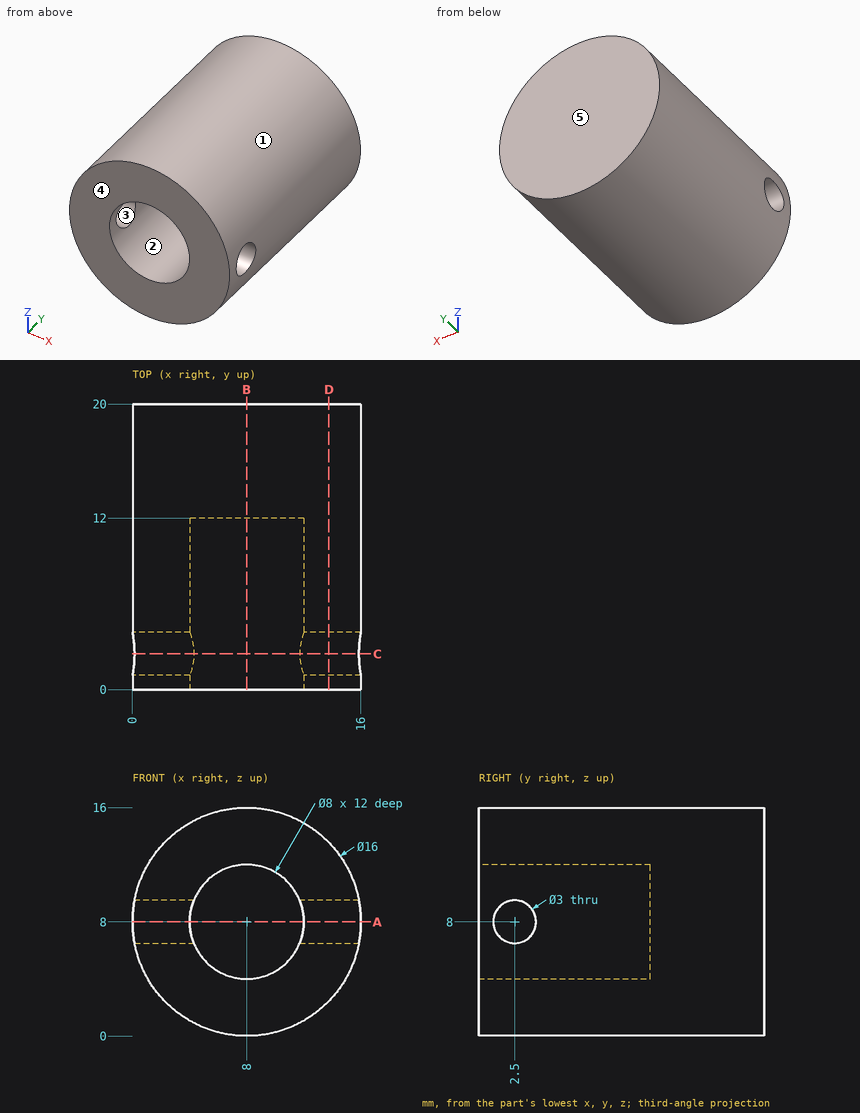
Here's the drawing with two shaded views (mm, measured from the low corner). I have some questions. A direction names the side the tool comes from. Give positions to 0.01 mm unless a question says otherwise; leave off trailing zeros. Loops run counter-clockwise (first coordinate to the right, second up) from the corner with the lowest first, then second, coordinate; pieces in that order, holes last. Notation, with made-up numbers: (-17, 58) -> (-8, 58) arc R26 ccw to (-8, 90) -> close; hole circle Ø8 at (-36, 20.25). An arc over 180 degrees is marked (long way). One line per item, written item: value.
Q1. Suppose I cut it at C-C on y = 2.5. Please give me the cut outline in (x, z).
Answers follow:
outline: (0.14, 6.5) arc R8 ccw to (15.86, 6.5) -> (11.71, 6.5) arc R4 cw to (4.29, 6.5) -> close; (0.14, 9.5) -> (4.29, 9.5) arc R4 cw to (11.71, 9.5) -> (15.86, 9.5) arc R8 ccw to start
Q2. On a 3-axis mill with a long thin cutter (end or side, diameter ignored), from which of +Z, -Z, +X, -X, +Y, -Y can I reach the whole of each face in a straight line? I mean the marked faces 1 and 2. Say none if no direction works.
Answers follow:
face 1: +Y, -Y
face 2: -Y
Q3. Suppose I cut it at A-A on z = 8. Please give me the cut outline in (x, y).
Answers follow:
outline: (0, 0) -> (4, 0) -> (4, 1) -> (0, 1) -> close; (0, 4) -> (4, 4) -> (4, 12) -> (12, 12) -> (12, 4) -> (16, 4) -> (16, 20) -> (0, 20) -> close; (12, 0) -> (16, 0) -> (16, 1) -> (12, 1) -> close
Q4. Suppose I cut it at D-D on x = 13.75. Please give me the cut outline in (y, z).
Answers follow:
outline: (0, 2.44) -> (20, 2.44) -> (20, 13.56) -> (0, 13.56) -> close; hole circle Ø3 at (2.5, 8)
Q5. I'm going to push flat-ended pins straight in: pin 1 Ø6 at (x, y) = (12, 8.5) entering from -Z; pin 2 Ø5 at (x, z) = (8, 8) entering from -Y; pin 3 Ø1 at (x, y) = (3.5, 3.5) entering from -Z. Where does each tip first touch, or does it pass through?
Answers follow:
pin 1: z = 0.06
pin 2: y = 12
pin 3: z = 1.07
Q6. We'd pull the mould along Y, two halves only. Please class the marked faces 3, 4 and 5: pulls with the +Y half, pulls with the -Y half, needs draft (parallel to the pull), parting line crosses it, or undercut.
Answers follow:
face 3: undercut
face 4: pulls with the -Y half
face 5: pulls with the +Y half
Q7. If I drill on line 1 along X through (y, z) = (6.5, 8); line 2 along Y through (x, z) = (2.7, 8); line 3 along X through (y, z) = (7.5, 5), over which ranges is the centre line in solid material (lowest first)?
Answers follow:
line 1: 0 to 4, 12 to 16
line 2: 0 to 1, 4 to 20
line 3: 0.58 to 5.35, 10.65 to 15.42
Q8. Suppose I cut it at B-B on x = 8. Please give me the cut outline in (y, z), then the cut area to 3 significant figures.
Answers follow:
outline: (0, 0) -> (20, 0) -> (20, 16) -> (0, 16) -> (0, 12) -> (12, 12) -> (12, 4) -> (0, 4) -> close
area: 224 mm^2
